Drawing for the job (mm, zero at the part's lowest x, y, z). A direction names the side the tool comes from. Round coordinates to 2 decimals unless told otherwise and drop trailing zeros. Loops run counter-clockwise (first coordinate to the right, second up) from the corner with the lowest first, then second, coordinate; pieces in that order, holes last.
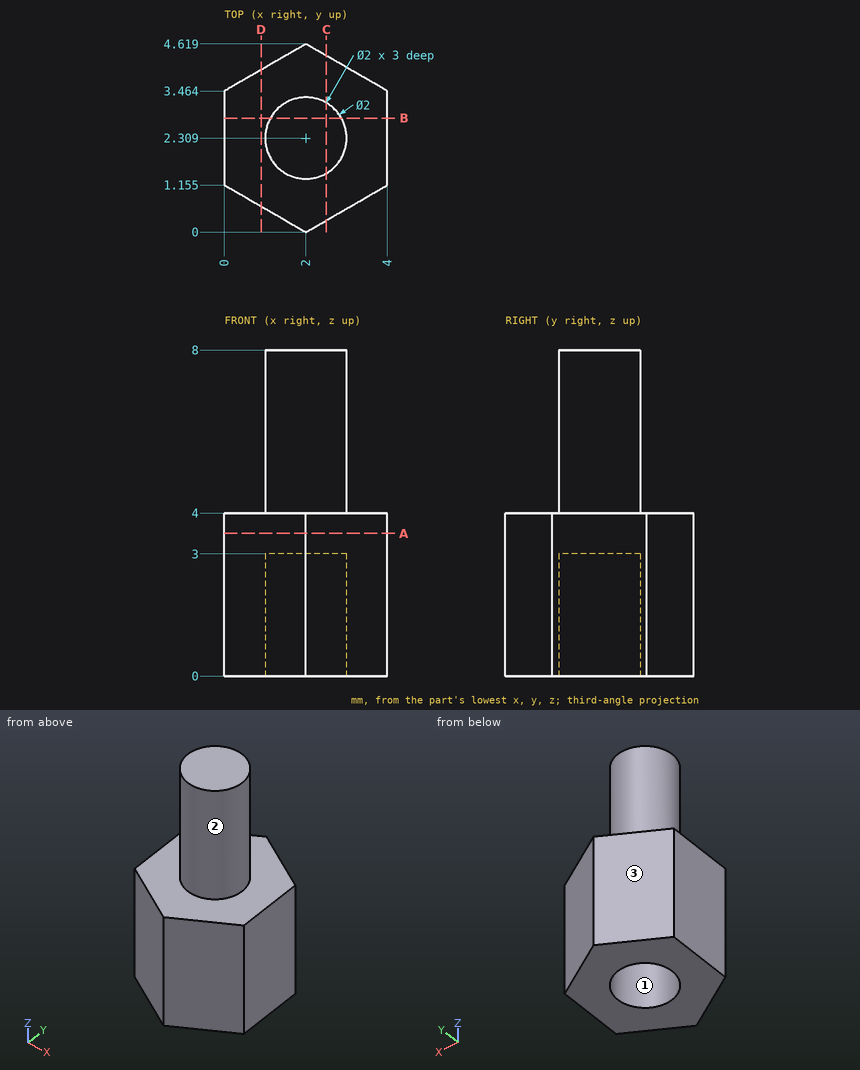
Q1. Slice it at A-A on z = 3.5. Give the cut face in (x, y) (1 decimal).
Q2. Slice it at D-D on x = 0.9. Give the cut face in (y, z) (1 decimal).
Q3. Probe line 1 (X direction, y = 2.25, z = 0.5); line 2 (Z direction, x = 3.2, y = 3.1); line 3 (Z direction, x = 1.4, y = 2.35). List the from-to ranges inside material, lowest first.
Q4. Tool access for the marked faces 1, 2 and 3: list every direction of +Z, -Z, +X, -X, +Y, -Y with a clear straight run to the whole face (end or side of a thin tool).
Q5. Slice it at C-C on x = 2.5. Give the cut face in (y, z) (1 decimal).
Q6. Slice it at B-B on y = 2.8. Give the cut face in (x, z).
Q7. Flat gauge pins, fed straight in: P1, Ø1.5, axis at y = 3.5, z = 4.5, coming from the +X side; P2, Ø2, axis at x = 3.5, z = 2.5, coming from the -Y side. Where does each tip first touch, or does it go through?
Reply:
1. outline: (0, 1.2) - (2, 0) - (4, 1.2) - (4, 3.5) - (2, 4.6) - (0, 3.5) - close
2. outline: (0.6, 0) - (4, 0) - (4, 4) - (0.6, 4) - close
3. line 1: x = 0 to 1, 3 to 4
3. line 2: z = 0 to 4
3. line 3: z = 3 to 8
4. face 1: -Z
4. face 2: +Z
4. face 3: +Z, -Z, -X, +Y
5. outline: (0.3, 0) - (1.4, 0) - (1.4, 3) - (3.2, 3) - (3.2, 0) - (4.3, 0) - (4.3, 4) - (3.2, 4) - (3.2, 8) - (1.4, 8) - (1.4, 4) - (0.3, 4) - close
6. outline: (0, 0) - (1.13, 0) - (1.13, 3) - (2.87, 3) - (2.87, 0) - (4, 0) - (4, 4) - (2.87, 4) - (2.87, 8) - (1.13, 8) - (1.13, 4) - (0, 4) - close
7. P1: stops at x = 4
7. P2: stops at y = 0.29
